```python
from build123d import *

# Parameters (mm, degrees)
ESQUISSE1_W        = 100
ESQUISSE1_H        = 100
ESQUISSE1_R        = 1.6
BOSS_EXTRU_1_DEPTH = 1.6
ESQUISSE2_R        = 11
BOSS_EXTRU_2_DEPTH = 52


with BuildPart() as part:
    # Esquisse1 → Boss.-Extru.1 (new body)
    with BuildSketch(Plane.XY):
        Rectangle(ESQUISSE1_W, ESQUISSE1_H)
        with Locations((-46, 46)):
            Circle(ESQUISSE1_R, mode=Mode.SUBTRACT)
        with Locations((46, 46)):
            Circle(ESQUISSE1_R, mode=Mode.SUBTRACT)
        with Locations((-46, -46)):
            Circle(ESQUISSE1_R, mode=Mode.SUBTRACT)
        with Locations((46, -46)):
            Circle(ESQUISSE1_R, mode=Mode.SUBTRACT)
    extrude(amount=BOSS_EXTRU_1_DEPTH)

    # Esquisse2 → Boss.-Extru.2 (add)
    with BuildSketch(Plane.XY.offset(1.6)):
        with Locations((-17.405055541, 34)):
            Circle(ESQUISSE2_R)
        with Locations((16.577398103, 34)):
            Circle(ESQUISSE2_R)
    extrude(amount=BOSS_EXTRU_2_DEPTH)


solid = part.part
```
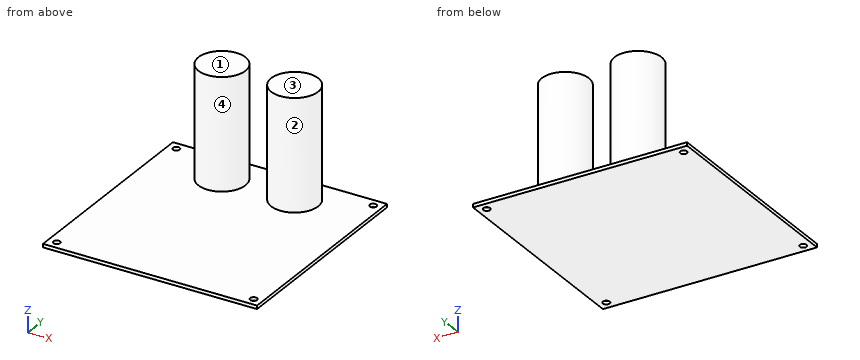
Check sheet for the modelled part. Datum: model origin and axes. Units: mm. Face numbers are marked on the shaded views. A direction names the side the tool comes from. Round coordinates to 2 decimals unless told otherwise and drop trailing zeros. Order: outer loops, then holes, each group sorted by start corner. A loop starts at its lowest first (then second) coordinate and runs counter-clockwise, first axis right, second up. Notation, with made-up numbers: (42, 34) - (77, 34) arc R24 ccw to (77, 62) - close; hole circle Ø5 at (54.5, -14). An arc over 180 degrees is marked (long way). Write item = value, one per line.
Q1. Go/stop test with flat-tipped pins: pin 1 (4 mm diameter, centred on x = 46, y = -46, fed in from +Z); pin 2 (4 mm diameter, centred on x = -27, z = 40.5, fed in from -Y); pin 3 (3 mm diameter, centred on x = -46, y = -46, fed in from +Z); pin 4 (10 mm diameter, centred on x = -32.5, z = 32, fed in from -Y). Record where each tip stops, or that it passes through.
Computed:
pin_1 = 1.6
pin_2 = 26.04
pin_3 = through
pin_4 = 29.63
Q2. Section check C-C (z = 22). Record the boundary of the cut face in (x, y), and give its area (3 significant figures).
Computed:
outline = circle Ø22 at (-17.41, 34); circle Ø22 at (16.58, 34)
area = 760 mm^2
Q3. Section check A-A (x = -46). Record the boundary of the cut face in (y, z).
Computed:
outline = (-50, 0) - (-47.6, 0) - (-47.6, 1.6) - (-50, 1.6) - close; (-44.4, 0) - (44.4, 0) - (44.4, 1.6) - (-44.4, 1.6) - close; (47.6, 0) - (50, 0) - (50, 1.6) - (47.6, 1.6) - close
Q4. Draft check along X on the marked faces 3 and 4. Enter one of: pulls with the +X half, pulls with the -X half, needs draft (parallel to the pull), parting line crosses it, or undercut.
Computed:
face_3 = needs draft
face_4 = undercut
Q5. Tool access check on the marked faces 1 and 2. Record the directions out of +Z, -Z, +X, -X, +Y, -Y that give a thin tool (end or side, any length) a straight path to the whole face; none if there is none.
Computed:
face_1 = +Z, +X, -X, +Y, -Y
face_2 = +Z
Q6. Section check D-D (x = 22). Record the boundary of the cut face in (y, z), and give its area (3 significant figures).
Computed:
outline = (-50, 0) - (50, 0) - (50, 1.6) - (43.57, 1.6) - (43.57, 53.6) - (24.43, 53.6) - (24.43, 1.6) - (-50, 1.6) - close
area = 1,160 mm^2
Q7. Thickness scan on line 1 along Y through (x, z) = (46, 0.9); line 2 along Z through (x, y) = (18, -8.5); line 3 along Y through (x, z) = (-13, 12). Record the ranges inside material, lowest first.
Computed:
line_1 = -50 to -47.6, -44.4 to 44.4, 47.6 to 50
line_2 = 0 to 1.6
line_3 = 23.92 to 44.08
